```python
from build123d import *

# Parameters (mm, degrees)
SKETCH1_W             = 50.8
SKETCH1_H             = 50.8
BOSS_EXTRUDE1_DEPTH   = 19.05
SKETCH1_3_W           = 12.7
SKETCH1_3_H           = 50.8
BOSS_EXTRUDE2_DEPTH   = 33.6804
M4X0_7_TAPPED_HOLE1_D = 3.3


with BuildPart() as part:
    # Sketch1 → Boss-Extrude1 (new body)
    with BuildSketch(Plane(origin=(0, 0, 0), x_dir=(1, 0, 0), z_dir=(0, 1, 0))):
        with Locations((6.35, 0)):
            Rectangle(SKETCH1_W, SKETCH1_H)
    extrude(amount=BOSS_EXTRUDE1_DEPTH)

    # Sketch1<3> → Boss-Extrude2 (add)
    with BuildSketch(Plane(origin=(0, 0, 0), x_dir=(1, 0, 0), z_dir=(0, 1, 0))):
        with Locations((-25.4, 0)):
            Rectangle(SKETCH1_3_W, SKETCH1_3_H)
    extrude(amount=BOSS_EXTRUDE2_DEPTH)

    # M4x0.7 Tapped Hole1 (through all)
    with Locations(Plane.ZY.offset(31.75)):
        with Locations((18, 30), (-18, 30)):
            Hole(M4X0_7_TAPPED_HOLE1_D / 2)


solid = part.part
```
Check sheet for the modelled part. Datum: model origin and axes. Units: mm. A direction names the side the tool comes from. Give positions to 0.01 mm unless a question says otherwise; leave off trailing zeros. Write each loop counter-clockwise with the first axis right and the second up, starting at its lowest first coordinate (ties: lowest second). Pieces come first, ordered by that corner, then holes. Notation, with made-up numbers: (71.5, 43) - (126.5, 43) arc R7 cw to (126.5, 55) - close; hole circle Ø11 at (-22.75, 19). An arc over 180 degrees is marked (long way). Answer as a JSON object with one key per item and string values. Group by question number.
1) Sectioned sample at D-D (y = 27). Record the cut outline in (x, z).
2) Sectioned sample at C-C (x = 22.5). Record the cut outline in (y, z), then the cut area to 3 significant figures.
3) Depth check by flat-ended pin: P1, Ø16, axis at y = 25.5, z = -3, coming from the +X side; P2, Ø2.5, axis at y = 30, z = 18, coming from the +X side; P3, Ø4, axis at y = 30, z = -18, coming from the +X side; P4, Ø6, axis at x = 13, z = 13.5, coming from the +Y side. Enter the tip coordinate at first touch or a pass-through.
4) Release check for a two-part mould opening along Y. For faces 3 (the face through (0, 0, 0)), 4 (the face through (-31.75, 17, 0)), 5 (the face through (-25.311, 31.636, -17.785)) record: pulls with the +Y half, pulls with the -Y half, needs draft (parallel to the pull), parting line crosses it, or undercut.
5) Sectioned sample at B-B (z = -3). Record the cut outline in (x, y), then the cut area to 3 significant figures.
6) Thickness scan on probe 1 along Y at (x, z) = (-23, -18); probe 2 along Y at (x, z) = (-10, 5); probe 3 along X at (y, z) = (23, 3.5). Record the ranges inside material, lowest first. Write a range as from..to.
7) Sectioned sample at A-A (z = 18). Record the cut outline in (x, y).
8) Access from +Z, -Z, +X, -X, +Y, -Y to the whole of each face (thin tool, end or side, straight path). Record for faces 1 (the face through (31.75, 9, 0)), 2 (the face through (6, 19.05, 0)).
Geometry results:
{
 "1": {"outline": "(-31.75, -25.4) - (-19.05, -25.4) - (-19.05, 25.4) - (-31.75, 25.4) - close"},
 "2": {"outline": "(0, -25.4) - (19.05, -25.4) - (19.05, 25.4) - (0, 25.4) - close", "area": "968 mm^2"},
 "3": {"P1": "stops at x = 31.75", "P2": "passes through", "P3": "stops at x = -19.05", "P4": "stops at y = 19.05"},
 "4": {"face 3": "pulls with the -Y half", "face 4": "needs draft", "face 5": "undercut"},
 "5": {"outline": "(-31.75, 0) - (31.75, 0) - (31.75, 19.05) - (-19.05, 19.05) - (-19.05, 33.68) - (-31.75, 33.68) - close", "area": "1,400 mm^2"},
 "6": {"probe 1": "y = 0..28.35, 31.65..33.68", "probe 2": "y = 0..19.05", "probe 3": "x = -31.75..-19.05"},
 "7": {"outline": "(-31.75, 0) - (31.75, 0) - (31.75, 19.05) - (-19.05, 19.05) - (-19.05, 28.35) - (-31.75, 28.35) - close; (-31.75, 31.65) - (-19.05, 31.65) - (-19.05, 33.68) - (-31.75, 33.68) - close"},
 "8": {"face 1": "+Z, -Z, +X, +Y, -Y", "face 2": "+Z, -Z, +X, +Y"}
}
